from build123d import *

# Parameters (mm, degrees)
SKETCH1_R                = 36.5
SKETCH1_R_2              = 4
BOSS_EXTRUDE1_DEPTH      = 145
BOSS_EXTRUDE2_DEPTH      = 170
BOSS_EXTRUDE2_DEPTH_BACK = 22
SKETCH1_3_R              = 4


with BuildPart() as part:
    # Sketch1 → Boss-Extrude1 (new body)
    with BuildSketch(Plane(origin=(0, 0, 0), x_dir=(0, 0, -1), z_dir=(1, 0, 0))):
        Circle(SKETCH1_R)
        Circle(SKETCH1_R_2, mode=Mode.SUBTRACT)
    extrude(amount=BOSS_EXTRUDE1_DEPTH)

    # Sketch1<3> → Boss-Extrude2 (add, two sides: drawn at the far end of the back side and taken through both)
    with BuildSketch(Plane(origin=(0, 0, 0), x_dir=(0, 0, -1), z_dir=(1, 0, 0)).offset(-BOSS_EXTRUDE2_DEPTH_BACK)):
        Circle(SKETCH1_3_R)
    extrude(amount=BOSS_EXTRUDE2_DEPTH + BOSS_EXTRUDE2_DEPTH_BACK)


solid = part.part
Source: CAD feature listing. Evaluate the final solid. Frame: model axes, mm. A direction names the side the tool comes from. Give positions to 0.01 mm unless a question says otherwise; leave off trailing zeros. Order: outer loops, then holes, each group sorted by start corner. A loop starts at its lowest first (then second) coordinate and runs counter-clockwise, first axis right, second up. Notation, with made-up numbers: (63.25, 49.25) -> (71.25, 49.25) arc R11 ccw to (71.25, 67.25) -> close; hole circle Ø8 at (-35, 36.25). An arc over 180 degrees is marked (long way). Write item = value, one per line.
Q1. Cut plane C-C, the plane x = 115.5. Output: boundary loops of the cut face in (y, z), and give its area (3 significant figures).
Data:
outline = circle Ø73 at (0, 0)
area = 4,190 mm^2
Q2. Cut plane A-A, the plane y = 0. Output: boundary loops of the cut face in (x, z).
Data:
outline = (-22, -4) -> (0, -4) -> (0, -36.5) -> (145, -36.5) -> (145, -4) -> (170, -4) -> (170, 4) -> (145, 4) -> (145, 36.5) -> (0, 36.5) -> (0, 4) -> (-22, 4) -> close
Q3. Cut plane D-D, the plane z = 12.5. Output: boundary loops of the cut face in (x, y), and give its area (3 significant figures).
Data:
outline = (0, -34.29) -> (145, -34.29) -> (145, 34.29) -> (0, 34.29) -> close
area = 9,940 mm^2
Q4. Pin query (flat end, axial travel): pin 1 (6 mm diameter, centred on y = -10.5, z = -18, fed in from +X); pin 2 (12 mm diameter, centred on x = 113, z = 11.5, fed in from +Y); pin 3 (6 mm diameter, centred on x = 116.5, y = 19, fed in from +Z). Return the tip coordinate at first contact, or that it passes through.
Data:
pin_1 = 145
pin_2 = 36.08
pin_3 = 32.81
Q5. Material intervals for line 1 (X direction, y = -23.5, z = 16.5); line 2 (Z direction, x = 125, y = 1); line 3 (Z direction, x = 29, y = -32), sorted ascending. Write a range as from..to.
Data:
line_1 = 0..145
line_2 = -36.49..36.49
line_3 = -17.56..17.56
Q6. Set-up query: faces 1 (the face through (170, 0, 0)), 2 (the face through (-11.154, -3.905, 0.867)), 3 (the face through (157.325, -3.905, 0.867)). Return all of +Z, -Z, +X, -X, +Y, -Y with unobstructed straight access to the full face (end or side cutting, diameter ignored); none if empty.
Data:
face_1 = +Z, -Z, +X, +Y, -Y
face_2 = -X
face_3 = +X
